from build123d import *

# Parameters (mm, degrees)
SKETCH5_W          = 15
SKETCH5_H          = 4
SKETCH7_R          = 2.5
CUT_EXTRUDE2_DEPTH = 5
FILLET1_R          = 2
SKETCH9_R          = 3.7
CUT_EXTRUDE3_DEPTH = 2.5
SKETCH6_R          = 2.5
CUT_EXTRUDE4_DEPTH = 5
SKETCH10_R         = 3.75
CUT_EXTRUDE5_DEPTH = 2.5


with BuildPart() as part:
    # Sweep1: sweep along a path in Sketch2
    with BuildLine(Plane.XY) as sweep1_path:
        Line((-25, 0), (-2.5, 0))
        ThreePointArc((-2.5, 0), (-0.732233047, 0.732233047), (0, 2.5))
        Line((0, 2.5), (0, 25))
    # Sketch5 → Sweep1 (sweep)
    with BuildSketch(Plane(origin=(-25, 0, 0), x_dir=(0, 0, -1), z_dir=(1, 0, 0))):
        Rectangle(SKETCH5_W, SKETCH5_H)
    sweep(path=sweep1_path.line)

    # Sketch7 → Cut-Extrude2 (cut, through all)
    with BuildSketch(Plane.ZY.offset(2)):
        with Locations((0, 17.5)):
            Circle(SKETCH7_R)
    extrude(amount=-CUT_EXTRUDE2_DEPTH, mode=Mode.SUBTRACT)

    # Fillet1
    fillet1_edges = [part.edges().sort_by_distance(p)[0] for p in [
        (-25, 0, 7.5),
        (0, 25, -7.5),
        (0, 25, 7.5),
        (-25, 0, -7.5),
    ]]
    fillet(fillet1_edges, radius=FILLET1_R)

    # Sketch9 → Cut-Extrude3 (cut)
    with BuildSketch(Plane.ZY.offset(2)):
        with Locations((0, 17.5)):
            Circle(SKETCH9_R)
    extrude(amount=-CUT_EXTRUDE3_DEPTH, mode=Mode.SUBTRACT)

    # Sketch6 → Cut-Extrude4 (cut, through all)
    with BuildSketch(Plane(origin=(0, 2, 0), x_dir=(1, 0, 0), z_dir=(0, 1, 0))):
        with Locations((-17.5, 0)):
            Circle(SKETCH6_R)
    extrude(amount=-CUT_EXTRUDE4_DEPTH, mode=Mode.SUBTRACT)

    # Sketch10 → Cut-Extrude5 (cut)
    with BuildSketch(Plane(origin=(0, 2, 0), x_dir=(1, 0, 0), z_dir=(0, 1, 0))):
        with Locations((-17.5, 0)):
            Circle(SKETCH10_R)
    extrude(amount=-CUT_EXTRUDE5_DEPTH, mode=Mode.SUBTRACT)


solid = part.part
CAD build for the part. Positions are in the model's coordinates, mm. A direction names the side the tool comes from. Give positions to 0.01 mm unless a question says otherwise; leave off trailing zeros. Loops run counter-clockwise (first coordinate to the right, second up) from the corner with the lowest first, then second, coordinate; pieces in that order, holes last. Notation, with made-up numbers: M 9,-29.5 L 46,-29.5 A14 ccw 46,-19.5 Z; hole C 79.5,30.25 d9. An arc over 180 degrees is marked long. Answer in a Markdown table with one row per item. Add a question column.
Item 1: Band-saw the part on C-C on z = 0. Give the cut face in (x, y), then the cut area to 3 significant figures.
Item 2: Band-saw the part on D-D on y = 0.5. Give the cut face in (x, z).
Item 3: Drop flat-ended pins along their axis: P1, Ø4.5, axis at y = 17.5, z = 0, coming from the +X side; P2, Ø8, axis at x = -17.5, z = 0, coming from the +Y side; P3, Ø2, axis at x = -18, z = -1.5, coming from the +Y side; P4, Ø6, axis at y = 11.5, z = -5.5, coming from the -X side. Give the stop position or say it passes through.
Item 4: Probe probe 1 along Y at (x, z) = (-10.75, -5.75); probe 2 along Z at (x, y) = (-17.5, -1.05). List the from-to ranges inside material, lowest first.
Item 5: Mould opens along Y. For faces 1 (the face through (-14, -2, 0)), 2 (the face through (-15, -0.5, 1)), 3 (the face through (-21.246, 0.768, -0.165)), 4 (the face through (0.5, 15, 1)) say: +Y half, -Y half, draft (parallel to the pull), parting line (faces both ways), or undercut.
Item 6: Tool access for faces 5 (the face through (-0.768, 13.888, -0.802)), 6 (the face through (-25, 0, 0)), 7 (the face through (-2, 14, -2)): list every direction of +Z, -Z, +X, -X, +Y, -Y with a clear straight run to the whole face (end or side of a thin tool).
Item 7: Band-saw the part on A-A on x = -17.5. Give the cut face in (y, z).
Item 8: Band-saw the part on B-B on y = 17.5. Give the cut face in (x, z), then the cut area to 3 significant figures.
Reply:
| question | item | result |
|---|---|---|
| 1 | outline | M -25,-2 L -20,-2 L -20,-0.5 L -21.25,-0.5 L -21.25,2 L -25,2 Z; M -15,-2 L -2.5,-2 A4.5 ccw 2,2.5 L 2,15 L 0.5,15 L 0.5,13.8 L -2,13.8 L -2,2.5 A0.5 cw -2.5,2 L -13.75,2 L -13.75,-0.5 L -15,-0.5 Z; M -2,21.2 L 0.5,21.2 L 0.5,20 L 2,20 L 2,25 L -2,25 Z |
| 1 | area | 143 mm^2 |
| 2 | outline | M -25,-5.5 A2 ccw -23,-7.5 L 1.53,-7.5 L 1.53,7.5 L -23,7.5 A2 ccw -25,5.5 Z; hole C -17.5,0 d7.5 |
| 3 | P1 | passes through |
| 3 | P2 | stops at y = 2 |
| 3 | P3 | stops at y = -0.5 |
| 3 | P4 | stops at x = -2 |
| 4 | probe 1 | y = -2 to 2 |
| 4 | probe 2 | z = -7.5 to -2.5, 2.5 to 7.5 |
| 5 | face 1 | -Y half |
| 5 | face 2 | +Y half |
| 5 | face 3 | draft |
| 5 | face 4 | undercut |
| 6 | face 5 | -X |
| 6 | face 6 | +Z, -Z, -X, +Y, -Y |
| 6 | face 7 | +Z, -Z, -X, +Y |
| 7 | outline | M -2,-7.5 L 2,-7.5 L 2,-3.75 L -0.5,-3.75 L -0.5,-2.5 L -2,-2.5 Z; M -2,2.5 L -0.5,2.5 L -0.5,3.75 L 2,3.75 L 2,7.5 L -2,7.5 Z |
| 8 | outline | M -2,-7.5 L 2,-7.5 L 2,-2.5 L 0.5,-2.5 L 0.5,-3.7 L -2,-3.7 Z; M -2,3.7 L 0.5,3.7 L 0.5,2.5 L 2,2.5 L 2,7.5 L -2,7.5 Z |
| 8 | area | 34.0 mm^2 |
